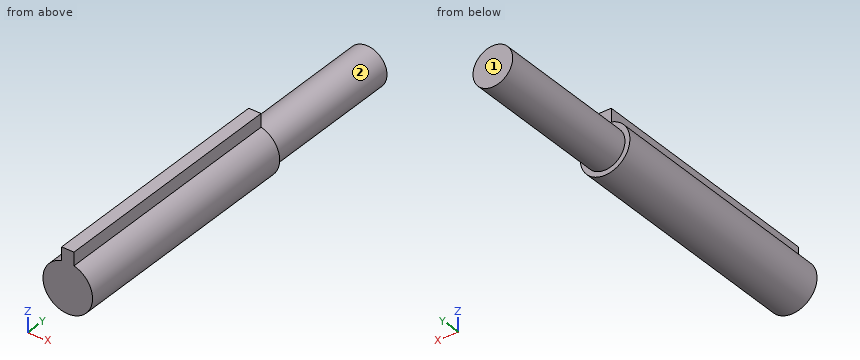
from build123d import *

# Parameters (mm, degrees)
SKETCH1_R           = 5
BOSS_EXTRUDE1_DEPTH = 50
SKETCH2_R           = 4
BOSS_EXTRUDE2_DEPTH = 30
SKETCH3_W           = 2.5
SKETCH3_H           = 5
BOSS_EXTRUDE3_DEPTH = 50


with BuildPart() as part:
    # Sketch1 → Boss-Extrude1 (new body)
    with BuildSketch(Plane(origin=(0, 0, 0), x_dir=(1, 0, 0), z_dir=(0, 1, 0))):
        Circle(SKETCH1_R)
    extrude(amount=BOSS_EXTRUDE1_DEPTH)

    # Sketch2 → Boss-Extrude2 (add)
    with BuildSketch(Plane(origin=(0, 50, 0), x_dir=(1, 0, 0), z_dir=(0, 1, 0))):
        Circle(SKETCH2_R)
    extrude(amount=BOSS_EXTRUDE2_DEPTH)

    # Sketch3 → Boss-Extrude3 (add)
    with BuildSketch(Plane.XZ):
        with Locations((0, 5)):
            Rectangle(SKETCH3_W, SKETCH3_H)
    extrude(amount=-BOSS_EXTRUDE3_DEPTH)


solid = part.part
Design review of the part built by this model. Coordinates are the model's own, in mm. Face numbers are marked on the shaded views. A direction names the side the tool comes from. Round coordinates to 2 decimals unless told otherwise and drop trailing zeros. Write each loop counter-clockwise with the first axis right and the second up, starting at its lowest first coordinate (ties: lowest second). Pieces come first, ordered by that corner, then holes.
Item 1: Consider section B-B on z = 0. Give the boundary of the cut face in (x, y).
Item 2: Consider section D-D on y = 29. Give the boundary of the cut face in (x, z).
Item 3: Consider section A-A on x = 0. Give the boundary of the cut face in (y, z).
Item 4: For pin 1 Ø2 at (y, z) = (58, 4) entering from -X; pin 2 Ø4 at (y, z) = (57.5, 5.5) entering from +X; pin 3 Ø3 at (y, z) = (27, 6.5) entering from +X, all flat-tipped, find the tip position at first contact; note any pin that passes through.
Item 5: Wall thickness on L1, parallel to X at y = 12, z = 6; L2, parallel to Y at x = -2.75, z = -3.25; L3, parallel to Z at x = 3, y = 8: over which ranges is each line inside the solid? List them lowest first.
Item 6: Consider section C-C on y = 58.5. Give the boundary of the cut face in (x, z), and give its area (3 significant figures).
Item 7: For the marked faces 1 and 2, list the 3-axis set-ups (+Z, -Z, +X, -X, +Y, -Y) from which the entire face can be reached by the end or side of a thin tool; tool diameter is ignored.
Check values:
1. outline: (-5, 0) - (5, 0) - (5, 50) - (4, 50) - (4, 80) - (-4, 80) - (-4, 50) - (-5, 50) - close
2. outline: (-1.25, 4.84) arc R5 ccw (long way) to (1.25, 4.84) - (1.25, 7.5) - (-1.25, 7.5) - close
3. outline: (0, -5) - (50, -5) - (50, -4) - (80, -4) - (80, 4) - (50, 4) - (50, 7.5) - (0, 7.5) - close
4. pin 1: stops at x = -2.65
4. pin 2: stops at x = 1.94
4. pin 3: stops at x = 1.25
5. L1: x = -1.25 to 1.25
5. L2: y = 0 to 50
5. L3: z = -4 to 4
6. outline: circle Ø8 at (0, 0)
6. area: 50.3 mm2
7. face 1: +Z, -Z, +X, -X, +Y
7. face 2: +Y
